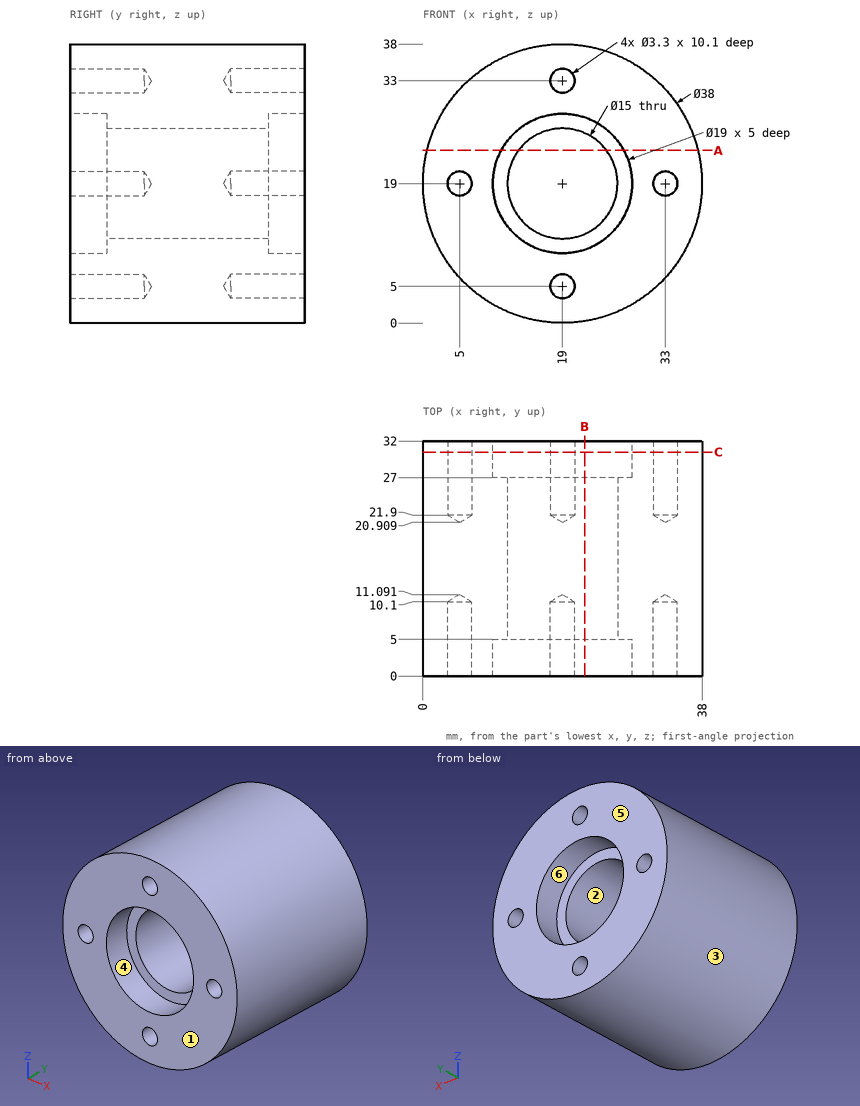
Check sheet for the drawn part. Datum: minimum x, y, z corner. Units: mm. A direction names the side the tool comes from. Give positions to 0.01 mm unless a question says otherwise; leave off trailing zeros. Write each loop counter-clockwise with the first axis right and the second up, starting at its lowest first coordinate (ties: lowest second). Pieces come first, ordered by that corner, then holes. Notation, with made-up numbers: (-8, 59) -> (7, 59) arc R12 cw to (7, 64) -> close; hole circle Ø2 at (24, 28). An arc over 180 degrees is marked (long way). Use one line per item in the form item = value. Start each with the question number.
1. Section check C-C (y = 30.5). Record the cut outline in (x, z).
2. Mould release check, pull along Z, two halves, no side actions. Record for the marked faces 1, 2 and 3: pulls with the +Z half, pulls with the -Z half, needs draft (parallel to the pull), parting line crosses it, or undercut.
3. Access from +Z, -Z, +X, -X, +Y, -Y to the whole of each face (thin tool, end or side, straight path). Record for the marked faces 4, 5 and 6.
4. Thickness scan on line 1 along X through (y, z) = (6.25, 19); line 2 along Y through (x, z) = (26.5, 14.5); line 3 along Z through (x, y) = (15, 10) (1 decimal). Record the ranges inside material, lowest first. Write a range as from..to.
5. Section check A-A (z = 23.5). Record the cut outline in (x, y), and give its area (3 significant figures).
6. Section check B-B (x = 22). Record the cut outline in (y, z), and give its area (3 significant figures).
7. Go/stop test with flat-tipped pins: P1, Ø3, axis at x = 19, z = 33, coming from the -Y side; P2, Ø2.5, axis at x = 19, z = 5, coming from the -Y side; P3, Ø8, axis at x = 5.5, y = 7, coming from the +Z side (1 decimal). Record where each tip stops, or that it passes through.
Conclusion:
q1.outline = circle Ø38 at (19, 19); hole circle Ø3.3 at (5, 19); hole circle Ø19 at (19, 19); hole circle Ø3.3 at (19, 5); hole circle Ø3.3 at (19, 33); hole circle Ø3.3 at (33, 19)
q2.face_1 = needs draft
q2.face_2 = undercut
q2.face_3 = parting line crosses it
q3.face_4 = -Y
q3.face_5 = +Z, -Z, +X, -X, +Y
q3.face_6 = +Y
q4.line_1 = 0..3.35, 6.65..11.5, 26.5..31.35, 34.65..38
q4.line_2 = 5..27
q4.line_3 = 0.4..12.7, 25.3..37.6
q5.outline = (0.54, 0) -> (10.63, 0) -> (10.63, 5) -> (13, 5) -> (13, 27) -> (10.63, 27) -> (10.63, 32) -> (0.54, 32) -> close; (25, 5) -> (27.37, 5) -> (27.37, 0) -> (37.46, 0) -> (37.46, 32) -> (27.37, 32) -> (27.37, 27) -> (25, 27) -> close
q5.area = 750 mm²
q6.outline = (0, 0.24) -> (32, 0.24) -> (32, 9.99) -> (27, 9.99) -> (27, 12.13) -> (5, 12.13) -> (5, 9.99) -> (0, 9.99) -> close; (0, 28.01) -> (5, 28.01) -> (5, 25.87) -> (27, 25.87) -> (27, 28.01) -> (32, 28.01) -> (32, 37.76) -> (0, 37.76) -> close
q6.area = 718 mm²
q7.P1 = 10.19
q7.P2 = 10.34
q7.P3 = 35.5
